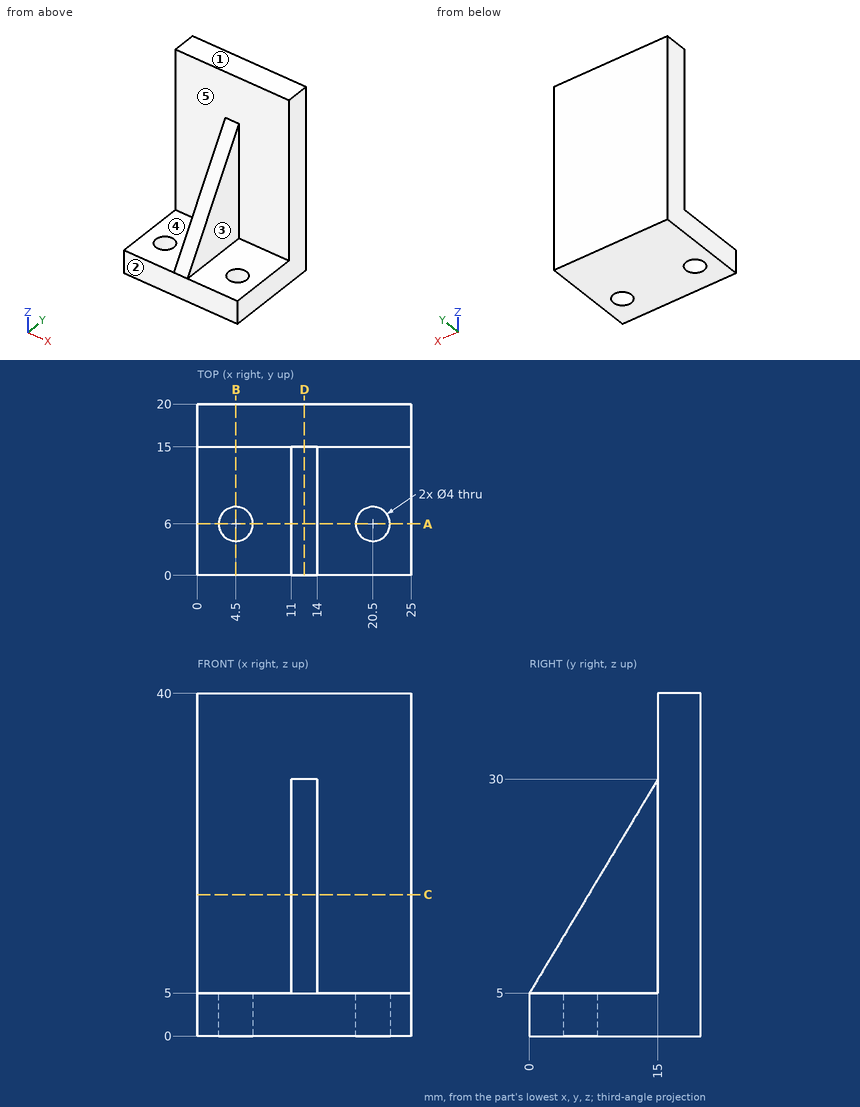
Verification items for this drawing (mm, ordinates from the low corner). A direction names the side the tool comes from. Coordinates: 2 decimals unless noted, no trailing zeros. Loops run counter-clockwise (first coordinate to the right, second up) from the corner with the lowest first, then second, coordinate; pieces in that order, holes last. Notation, with made-up numbers: (55, 79.5) -> (98, 79.5) arc R8 cw to (98, 86.5) -> close; hole circle Ø2 at (13, 38). An arc over 180 degrees is marked (long way). Answer in a Markdown table with one row per item. Add a question column.
1. Section check A-A, the plane y = 6. Enter the section's corners in (x, z).
2. Material ranges on probe 1 along Y at (x, z) = (20.5, 2.8); probe 2 along Y at (x, z) = (19.5, 16); probe 3 along Z at (x, y) = (19.5, 1.5), recorded low to high. Write a range as [from, to].
3. Section check D-D, the plane x = 12.5. Enter the section's corners in (y, z), then the cut area to 4 significant figures.
4. Access from +Z, -Z, +X, -X, +Y, -Y to the whole of each face (thin tool, end or side, straight path). Record for the marked faces 1, 2, 3, 4 and 5.
5. Section check B-B, the plane x = 4.5. Enter the section's corners in (y, z).
6. Depth check by flat-ended pin: P1, Ø1.5, axis at y = 10, z = 9, coming from the +X side; P2, Ø4.5, axis at y = 9.5, z = 22, coming from the -X side; P3, Ø9, axis at x = 20.5, y = 8.5, coming from the +Z side. Enter the tip coordinate at first touch or a pass-through.
7. Section check C-C, the plane z = 16.5. Enter the section's corners in (x, y).
Derived:
| question | item | result |
|---|---|---|
| 1 | outline | (0, 0) -> (2.5, 0) -> (2.5, 5) -> (0, 5) -> close; (6.5, 0) -> (18.5, 0) -> (18.5, 5) -> (14, 5) -> (14, 15) -> (11, 15) -> (11, 5) -> (6.5, 5) -> close; (22.5, 0) -> (25, 0) -> (25, 5) -> (22.5, 5) -> close |
| 2 | probe 1 | y = [0, 4], [8, 20] |
| 2 | probe 2 | y = [15, 20] |
| 2 | probe 3 | z = [0, 5] |
| 3 | outline | (0, 0) -> (20, 0) -> (20, 40) -> (15, 40) -> (15, 30) -> (0, 5) -> close |
| 3 | area | 462.5 mm² |
| 4 | face 1 | +Z, +X, -X, +Y, -Y |
| 4 | face 2 | +Z, -Z, +X, -X, -Y |
| 4 | face 3 | +Z, +X, -Y |
| 4 | face 4 | +Z, -X, -Y |
| 4 | face 5 | +Z, -Y |
| 5 | outline | (0, 0) -> (4, 0) -> (4, 5) -> (0, 5) -> close; (8, 0) -> (20, 0) -> (20, 40) -> (15, 40) -> (15, 5) -> (8, 5) -> close |
| 6 | P1 | stops at x = 14 |
| 6 | P2 | stops at x = 11 |
| 6 | P3 | stops at z = 5 |
| 7 | outline | (0, 15) -> (11, 15) -> (11, 6.9) -> (14, 6.9) -> (14, 15) -> (25, 15) -> (25, 20) -> (0, 20) -> close |
